Source: three-view drawing plus pictorial views. Frame: mm from the lowest corner of the part. A direction names the side the tool comes from. Give positions to 0.01 mm unless a question says otherwise; leave off trailing zeros. Loops run counter-clockwise (first coordinate to the right, second up) from the corner with the lowest first, then second, coordinate; pieces in that order, holes last. Notation, with made-up numbers: M 44.25,-8.5 L 93.25,-8.5 A35 ccw 93.25,23.5 Z; hole C -21,52 d2. An arc over 180 degrees is marked long. Write item = value, one per line.
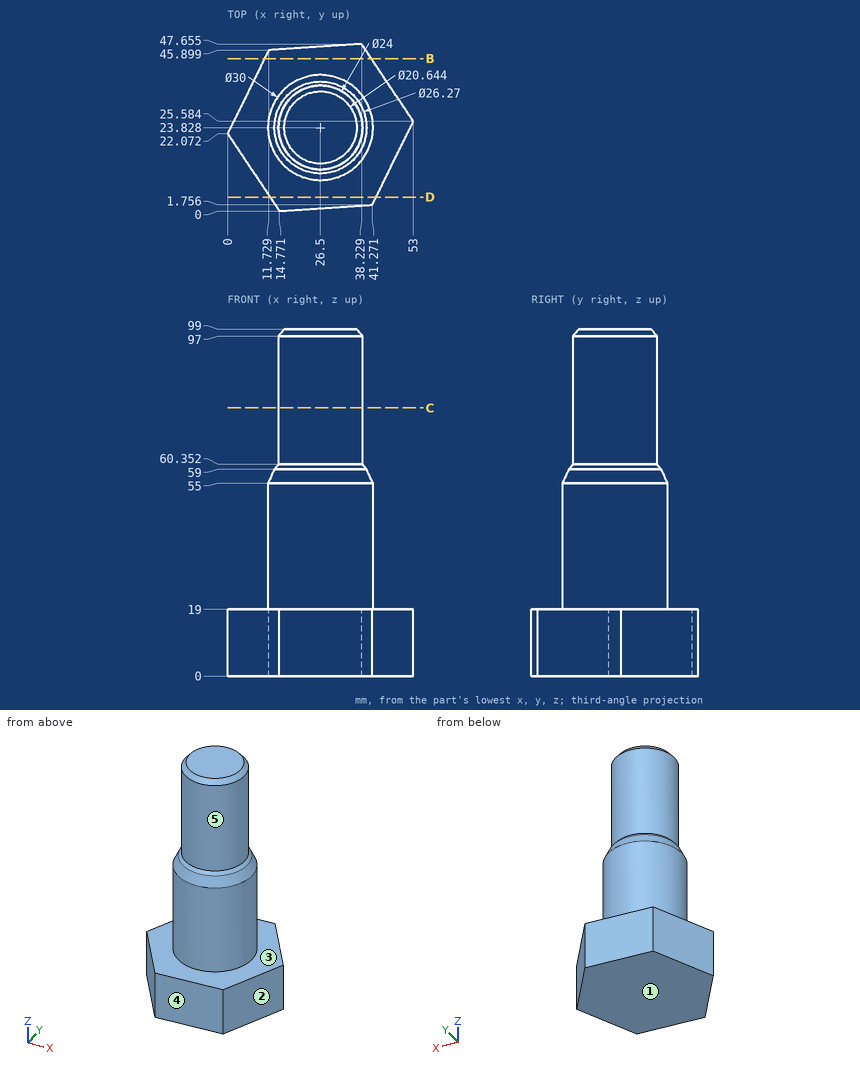
1. Cut plane B-B, the plane y = 43.5. Return the cut outline in (x, z).
Derived:
outline = M 10.55,0 L 41.01,0 L 41.01,19 L 10.55,19 Z
2. Material intervals for probe 1 along Y at (x, z) = (26, 95); probe 2 along Z at (x, y) = (14.5, 10); probe 3 along Y at (x, z) = (41.5, 7) (1 decimal), sorted ascending. Write a range as from..to.
Derived:
probe_1 = 11.84..35.82
probe_2 = 0..19
probe_3 = 2.2..42.8
3. Reachability of the marked faces 4 and 5 from +Z, -Z, +X, -X, +Y, -Y: full face, straight path, thin tool, end or side. Return the list, or none.
Derived:
face_4 = +Z, -Z, +X, -Y
face_5 = +Z
4. Pull-direction query (Z, two-part tool) for the marked faces 1, 2 and 3; classes: +Z half, -Z half, draft (parallel to the pull), parting line (faces both ways), or undercut.
Derived:
face_1 = -Z half
face_2 = draft
face_3 = +Z half
5. First-contact query: pin 1 Ø24 at (x, y) = (18.5, 15.5) entering from +Z; pin 2 Ø10 at (x, z) = (21.5, 72.5) entering from +Y; pin 3 Ø1 at (x, z) = (32.5, 37) entering from -Y; pin 4 Ø6 at (x, z) = (42.5, 23) entering from +Y. Flat tips, straight axial feed; report the tip coordinate or a pass-through.
Derived:
pin_1 = 99
pin_2 = 35.83
pin_3 = 9.87
pin_4 = 31.31
6. Cut plane D-D, the plane y = 4. Return the cut outline in (x, z) (1 decimal).
Derived:
outline = M 12.1,0 L 42.4,0 L 42.4,19 L 12.1,19 Z
7. Cut plane C-C, the plane z = 76.5. Return the cut outline in (x, y), then the cut area to 3 significant figures.
Derived:
outline = C 26.5,23.83 d24
area = 452 mm²
